Part model, mm, in its own coordinate system. Face numbers are marked on the shaded views. Coordinates: 2 decimals unless noted, no trailing zeros. Loops run counter-clockwise (first coordinate to the right, second up) from the corner with the lowest first, then second, coordinate; pieces in that order, holes last.
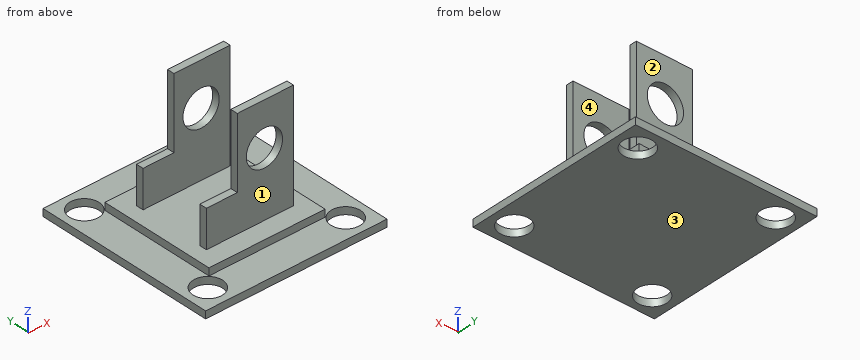
Autodesk Inventor part; units mm, degrees
ref_plane "YZ Plane" through (0, 0, 0) normal (1, 0, 0) x (0, 1, 0)
ref_plane "XZ Plane" through (0, 0, 0) normal (0, 1, 0) x (-1, 0, 0)
ref_plane "XY Plane" through (0, 0, 0) normal (0, 0, 1) x (1, 0, 0)
sketch "Sketch1" plane through (0, 0, 0) normal (0, 0, 1) x (1, 0, 0)
  line L0 (15.875, 15.875) -> (-15.875, 15.875)
  line L1 (-15.875, 15.875) -> (-15.875, -15.875)
  line L2 (-15.875, -15.875) -> (15.875, -15.875)
  line L3 (15.875, -15.875) -> (15.875, 15.875)
  line L4 (15.875, 15.875) -> (-15.875, -15.875) construction
  line L5 (-15.875, 15.875) -> (15.875, -15.875) construction
  point P0 (0, 0)
  dimension "d0" = 31.75
  dimension "d1" = 31.75
extrude "Extrusion1" add sketch "Sketch1" along normal blind 1.27
sketch "Sketch2" plane through (0, 0, 1.27) normal (0, 0, 1) x (1, 0, 0)
  line L0 (-10.16, 10.16) -> (10.16, 10.16)
  line L1 (10.16, 10.16) -> (10.16, -10.16)
  line L2 (10.16, -10.16) -> (-10.16, -10.16)
  line L3 (-10.16, -10.16) -> (-10.16, 10.16)
  line L4 (15.875, 15.875) -> (-15.875, 15.875)
  line L5 (15.875, -15.875) -> (15.875, 15.875)
  line L6 (-15.875, -15.875) -> (15.875, -15.875)
  line L7 (-15.875, 15.875) -> (-15.875, -15.875)
  point P0 (0, 0)
  dimension "d4" = 5.715
  dimension "d5" = 5.715
  dimension "d6" = 5.715
  dimension "d7" = 5.715
extrude "Extrusion2" add sketch "Sketch2" along normal blind 1.27 contours L0 L1 L2 L3
sketch "Sketch3" plane through (0, 0, 2.54) normal (0, 0, 1) x (1, 0, 0)
  line L0 (-7.62, 5.5499) -> (7.62, 5.5499)
  line L1 (7.62, 5.5499) -> (7.62, 6.8199)
  line L2 (7.62, 6.8199) -> (-7.62, 6.8199)
  line L3 (-7.62, 6.8199) -> (-7.62, 5.5499)
  line L4 (10.16, -10.16) -> (10.16, 10.16)
  line L5 (-10.16, 10.16) -> (-10.16, -10.16)
  line L6 (10.16, 10.16) -> (-10.16, 10.16)
  line L7 (-7.62, -6.8199) -> (7.62, -6.8199)
  line L8 (7.62, -6.8199) -> (7.62, -5.5499)
  line L9 (7.62, -5.5499) -> (-7.62, -5.5499)
  line L10 (-7.62, -5.5499) -> (-7.62, -6.8199)
  line L11 (-10.16, -10.16) -> (10.16, -10.16)
  point P0 (0, 0)
  dimension "d49" = 11.0998
  dimension "d50" = 1.27
  dimension "d60" = 1.27
  dimension "d61" = 5.5499
extrude "Extrusion3" add sketch "Sketch3" along normal blind 19.05 contours L3 L2 L1 L0 | L10 L9 L8 L7
sketch "Sketch4" plane through (-7.62, -6.8199, 2.54) normal (0, -1, 0) x (1, 0, 0)
  circle A0 centre (10.16, 11.43) radius 3.175
  line L0 (0, 19.05) -> (15.24, 19.05)
  line L1 (0, 0) -> (0, 19.05)
  point P0 (7.62, -2.54)
  dimension "d20" = 6.35
  dimension "d21" = 7.62
  dimension "d44" = 10.16
extrude "Extrusion4" cut sketch "Sketch4" against normal blind 127
sketch "Sketch5" plane through (0, 0, 1.27) normal (0, 0, 1) x (1, 0, 0)
  circle A0 centre (-12.065, 12.065) radius 2.5797
  line L0 (-15.875, -15.875) -> (15.875, -15.875)
  line L1 (15.875, -15.875) -> (15.875, 15.875)
  circle A1 centre (12.065, 12.065) radius 2.5797
  line L2 (15.875, 15.875) -> (-15.875, 15.875)
  line L3 (-15.875, 15.875) -> (-15.875, -15.875)
  circle A2 centre (-12.065, -12.065) radius 2.5797
  circle A3 centre (12.065, -12.065) radius 2.5797
  point P0 (0, 0)
  dimension "d24" = 5.1594
  dimension "d28" = 5.1594
  dimension "d29" = 3.81
  dimension "d30" = 3.81
  dimension "d31" = 3.81
  dimension "d32" = 3.81
  dimension "d33" = 5.1594
  dimension "d34" = 3.81
  dimension "d35" = 3.81
  dimension "d36" = 5.1594
  dimension "d37" = 3.81
  dimension "d38" = 3.81
extrude "Extrusion5" cut sketch "Sketch5" against normal blind 12.7 contours A0 | A1 | A2 | A3
sketch "Sketch6" plane through (-7.62, -6.8199, 2.54) normal (0, -1, 0) x (1, 0, 0)
  line L0 (0, 0) -> (0, 19.05)
  line L1 (0, 19.05) -> (15.24, 19.05)
  line L2 (0, 6.5528) -> (5.4184, 6.5528)
  line L3 (5.4184, 6.5528) -> (5.4184, 19.05)
  line L4 (5.4184, 19.05) -> (0, 19.05)
  line L5 (0, 19.05) -> (0, 6.5528)
  point P0 (7.62, -2.54)
extrude "Extrusion6" cut sketch "Sketch6" against normal blind 101.6
equation "\"d5\" = d4"
equation "\"d6\" = d4"
equation "\"d7\" = d4"
equation "\"d50\" = d60"
equation "\"d28\" = d24"
equation "\"d30\" = d29"
equation "\"d31\" = d29"
equation "\"d32\" = d29"
equation "\"d33\" = d24"
equation "\"d34\" = d29"
equation "\"d35\" = d29"
equation "\"d36\" = d24"
equation "\"d37\" = d29"
equation "\"d38\" = d29"
properties part number "pneumatics back holder"
Q1. Mould opens along Y. For the marked faces 1, 2, 3 and 4 say: released by +Y, released by -Y, zero draft, split by the parting line, or undercut.
Q2. Saw through at B-B (x = 2.54). List the corners of the cut face in (y, z) (3 decimals), plus the area to 3 significant figures.
Q3. Saw through at C-C (z = 13.97). List the corners of the cut face in (x, y) (3 decimals), plus the area to 3 significant figures.
Q4. Drop flat-ended pins along their axis: P1, Ø8, axis at x = 4.5, y = -1, coming from the +Z side; P2, Ø1, axis at y = 0, z = 2, coming from the +X side; P3, Ø8.5, axis at x = 2.54, z = 13.97, coming from the +Y side; P4, Ø4, axis at x = 12.065, y = 12.065, coming from the -Z side. Give the stop position or say it passes through.
Q5. Saw through at D-D (x = -9). List the corners of the cut face in (y, z) (3 decimals), plus the area to 3 significant figures.
Q6. Saw through at A-A (z = 6.5). List the corners of the cut face in (x, y), plus the area to 3 significant figures.
Q7. Probe line 1 (Y direction, x = 2, z = 10.5); line 2 (Z direction, x = 2.54, y = 6.15) (3 decimals); line 3 (Z direction, x = 12, y = -5). List the from-to ranges inside material, lowest first.
Checked values:
1. face 1: released by -Y
1. face 2: released by +Y
1. face 3: zero draft
1. face 4: undercut
2. outline: (-15.875, 0) - (15.875, 0) - (15.875, 1.27) - (10.16, 1.27) - (10.16, 2.54) - (6.82, 2.54) - (6.82, 10.795) - (5.55, 10.795) - (5.55, 2.54) - (-5.55, 2.54) - (-5.55, 10.795) - (-6.82, 10.795) - (-6.82, 2.54) - (-10.16, 2.54) - (-10.16, 1.27) - (-15.875, 1.27) - close; (-6.82, 17.145) - (-5.55, 17.145) - (-5.55, 21.59) - (-6.82, 21.59) - close; (5.55, 17.145) - (6.82, 17.145) - (6.82, 21.59) - (5.55, 21.59) - close
2. area: 98.4 mm2
3. outline: (-2.202, -6.82) - (-0.635, -6.82) - (-0.635, -5.55) - (-2.202, -5.55) - close; (-2.202, 5.55) - (-0.635, 5.55) - (-0.635, 6.82) - (-2.202, 6.82) - close; (5.715, -6.82) - (7.62, -6.82) - (7.62, -5.55) - (5.715, -5.55) - close; (5.715, 5.55) - (7.62, 5.55) - (7.62, 6.82) - (5.715, 6.82) - close
3. area: 8.82 mm2
4. P1: stops at z = 2.54
4. P2: stops at x = 10.16
4. P3: stops at y = 6.82
4. P4: passes through
5. outline: (-15.875, 0) - (15.875, 0) - (15.875, 1.27) - (10.16, 1.27) - (10.16, 2.54) - (-10.16, 2.54) - (-10.16, 1.27) - (-15.875, 1.27) - close
5. area: 66.1 mm2
6. outline: (-7.62, -6.82) - (7.62, -6.82) - (7.62, -5.55) - (-7.62, -5.55) - close; (-7.62, 5.55) - (7.62, 5.55) - (7.62, 6.82) - (-7.62, 6.82) - close
6. area: 38.7 mm2
7. line 1: y = -6.82 to -5.55, 5.55 to 6.82
7. line 2: z = 0 to 10.795, 17.145 to 21.59
7. line 3: z = 0 to 1.27
